CAD build for the part. Positions are in the model's coordinates, mm. Face numbers are marked on the shaded views. A direction names the side the tool comes from. Give positions to 0.01 mm unless a question says otherwise; leave off trailing zeros. Loops run counter-clockwise (first coordinate to the right, second up) from the corner with the lowest first, then second, coordinate; pieces in that order, holes last.
Item 1: Saw through at B-B on z = 1.25. Give the cut face in (x, y).
Item 2: Mould opens along X. For the marked faces 1, 2, 3 and 4 say: released by +X, released by -X, zero draft, split by the parting line, or undercut.
Item 3: Which spindle directions (+Z, -Z, +X, -X, +Y, -Y) get a long thin tool onto all of the face, cutting with end or side? Do the marked faces 5 and 6. Say none if no direction does.
Item 4: Saw through at D-D on y = -15. Give the cut face in (x, z).
Item 5: Probe probe 1 along X at (y, z) = (-1, 9); probe 2 along Y at (x, z) = (0, 10); probe 3 along Z at (x, y) = (1.5, -7.5). List the from-to ranges inside material, lowest first.
Item 6: Saw through at A-A on y = 0. Give the cut face in (x, z).
Item 7: Saw through at C-C on x = 3. Give the cut face in (y, z), plus the area to 3 significant figures.
Item 8: Drop flat-ended pins along their axis: P1, Ø5, axis at y = -16, z = 9.5, coming from the -X side; P2, Ø12, axis at y = -7.5, z = -9, coming from the +X side; P3, Ø2.5, axis at x = -13.75, y = 0, coming from the +Z side; P4, Ø6, axis at x = -2.5, z = 2.5, coming from the -Y side. Give the stop position or say it passes through.
from build123d import *

# Parameters (mm, degrees)
SKETCH1_R           = 17.5
SKETCH1_R_2         = 5
SKETCH1_R_3         = 1.5
BOSS_EXTRUDE1_DEPTH = 13.5
BOSS_EXTRUDE2_START = -7
SKETCH2_R           = 22.5
SKETCH2_R_2         = 17.5
BOSS_EXTRUDE2_DEPTH = 7
SKETCH3_R           = 7.5
SKETCH3_R_2         = 5
BOSS_EXTRUDE3_DEPTH = 8.5
SKETCH4_R           = 9
CUT_EXTRUDE1_DEPTH  = 8


with BuildPart() as part:
    # Sketch1 → Boss-Extrude1 (new, symmetric)
    with BuildSketch(Plane.XY):
        Circle(SKETCH1_R)
        Circle(SKETCH1_R_2, mode=Mode.SUBTRACT)
        with Locations((-13.75, 0)):
            Circle(SKETCH1_R_3, mode=Mode.SUBTRACT)
        with Locations((13.75, 0)):
            Circle(SKETCH1_R_3, mode=Mode.SUBTRACT)
    extrude(amount=BOSS_EXTRUDE1_DEPTH, both=True)

    # Sketch2 → Boss-Extrude2 (add)
    with BuildSketch(Plane(origin=(0, 0, -13.5), x_dir=(-1, 0, 0), z_dir=(0, 0, -1)).offset(BOSS_EXTRUDE2_START)):
        Circle(SKETCH2_R)
        Circle(SKETCH2_R_2, mode=Mode.SUBTRACT)
    extrude(amount=BOSS_EXTRUDE2_DEPTH)

    # Sketch3 → Boss-Extrude3 (add, symmetric)
    with BuildSketch(Plane.XY):
        Circle(SKETCH3_R)
        Circle(SKETCH3_R_2, mode=Mode.SUBTRACT)
    extrude(amount=BOSS_EXTRUDE3_DEPTH, both=True)

    # Sketch4 → Cut-Extrude1 (cut)
    with BuildSketch(Plane.XY.offset(13.5)):
        Circle(SKETCH4_R)
    extrude(amount=-CUT_EXTRUDE1_DEPTH, mode=Mode.SUBTRACT)


solid = part.part
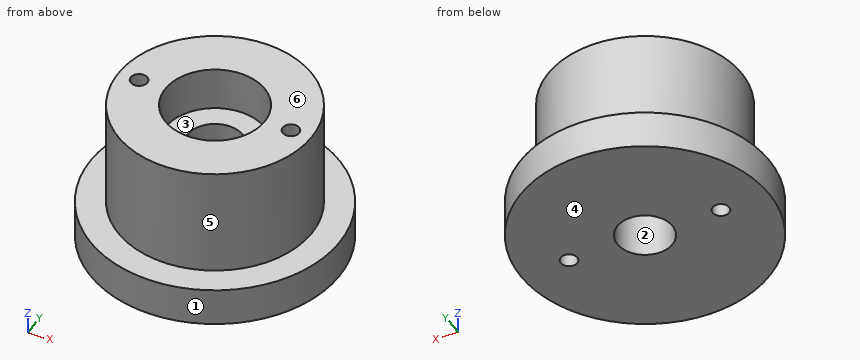
Results below:
1. outline: circle Ø35 at (0, 0); hole circle Ø3 at (-13.75, 0); hole circle Ø10 at (0, 0); hole circle Ø3 at (13.75, 0)
2. face 1: split by the parting line
2. face 2: undercut
2. face 3: undercut
2. face 4: zero draft
3. face 5: +Z
3. face 6: +Z, +X, -X, +Y, -Y
4. outline: (-16.77, -13.5) - (16.77, -13.5) - (16.77, -6.5) - (9.01, -6.5) - (9.01, 13.5) - (-9.01, 13.5) - (-9.01, -6.5) - (-16.77, -6.5) - close
5. probe 1: x = -17.47 to -14.87, -12.63 to -8.94, 8.94 to 12.63, 14.87 to 17.47
5. probe 2: y = -17.5 to -9, 9 to 17.5
5. probe 3: z = -13.5 to 5.5
6. outline: (-22.5, -13.5) - (-15.25, -13.5) - (-15.25, 13.5) - (-17.5, 13.5) - (-17.5, -6.5) - (-22.5, -6.5) - close; (-12.25, -13.5) - (-5, -13.5) - (-5, 5.5) - (-9, 5.5) - (-9, 13.5) - (-12.25, 13.5) - close; (5, -13.5) - (12.25, -13.5) - (12.25, 13.5) - (9, 13.5) - (9, 5.5) - (5, 5.5) - close; (15.25, -13.5) - (22.5, -13.5) - (22.5, -6.5) - (17.5, -6.5) - (17.5, 13.5) - (15.25, 13.5) - close
7. outline: (-22.3, -13.5) - (-4, -13.5) - (-4, 5.5) - (-8.49, 5.5) - (-8.49, 13.5) - (-17.24, 13.5) - (-17.24, -6.5) - (-22.3, -6.5) - close; (4, -13.5) - (22.3, -13.5) - (22.3, -6.5) - (17.24, -6.5) - (17.24, 13.5) - (8.49, 13.5) - (8.49, 5.5) - (4, 5.5) - close
7. area: 714 mm2
8. P1: stops at x = -11.14
8. P2: stops at x = 22.45
8. P3: passes through
8. P4: stops at y = -17.5
